```python
from build123d import *

# Parameters (mm, degrees)
SKETCH2_W           = 98
SKETCH2_H           = 42
SKETCH2_R           = 6
BOSS_EXTRUDE1_DEPTH = 20
SKETCH3_W           = 70
SKETCH3_H           = 6
CUT_EXTRUDE2_DEPTH  = 20
SKETCH4_W           = 70
SKETCH4_H           = 6
CUT_EXTRUDE3_DEPTH  = 20
SKETCH5_W           = 4.083920217
SKETCH5_H           = 6
CUT_EXTRUDE4_DEPTH  = 20
SKETCH6_W           = 4.083920217
SKETCH6_H           = 6
CUT_EXTRUDE5_DEPTH  = 20
SKETCH7_W           = 38.167840434
SKETCH7_H           = 6
CUT_EXTRUDE6_DEPTH  = 20
SKETCH8_R           = 10
BOSS_EXTRUDE2_DEPTH = 7
FILLET2_R           = 5
FILLET3_R           = 10


with BuildPart() as part:
    # Sketch2 → Boss-Extrude1 (new body)
    with BuildSketch(Plane(origin=(0, 0, 0), x_dir=(1, 0, 0), z_dir=(0, 1, 0))):
        Rectangle(SKETCH2_W, SKETCH2_H)
        with Locations((25, 0)):
            Circle(SKETCH2_R, mode=Mode.SUBTRACT)
        with Locations((-25, 0)):
            Circle(SKETCH2_R, mode=Mode.SUBTRACT)
    extrude(amount=-BOSS_EXTRUDE1_DEPTH)

    # Sketch3 → Cut-Extrude2 (cut)
    with BuildSketch(Plane.XY.offset(21)):
        with Locations((0, -17)):
            Rectangle(SKETCH3_W, SKETCH3_H)
    extrude(amount=-CUT_EXTRUDE2_DEPTH, mode=Mode.SUBTRACT)

    # Sketch4 → Cut-Extrude3 (cut)
    with BuildSketch(Plane(origin=(0, 0, -21), x_dir=(-1, 0, 0), z_dir=(0, 0, -1))):
        with Locations((0, -17)):
            Rectangle(SKETCH4_W, SKETCH4_H)
    extrude(amount=-CUT_EXTRUDE3_DEPTH, mode=Mode.SUBTRACT)

    # Sketch5 → Cut-Extrude4 (cut)
    with BuildSketch(Plane.XY.offset(1)):
        with Locations((32.958039892, -17)):
            Rectangle(SKETCH5_W, SKETCH5_H)
    extrude(amount=-CUT_EXTRUDE4_DEPTH, mode=Mode.SUBTRACT)

    # Sketch6 → Cut-Extrude5 (cut)
    with BuildSketch(Plane.XY.offset(1)):
        with Locations((-32.958039892, -17)):
            Rectangle(SKETCH6_W, SKETCH6_H)
    extrude(amount=-CUT_EXTRUDE5_DEPTH, mode=Mode.SUBTRACT)

    # Sketch7 → Cut-Extrude6 (cut)
    with BuildSketch(Plane.XY.offset(1)):
        with Locations((0, -17)):
            Rectangle(SKETCH7_W, SKETCH7_H)
    extrude(amount=-CUT_EXTRUDE6_DEPTH, mode=Mode.SUBTRACT)

    # Sketch8 → Boss-Extrude2 (add, symmetric)
    with BuildSketch(Plane.ZY):
        with BuildLine():
            Line((-21, 0), (21, 0))
            Line((21, 0), (21, 21))
            ThreePointArc((21, 21), (0, 42), (-21, 21))
            Line((-21, 21), (-21, 0))
        make_face()
        with Locations((0, 21)):
            Circle(SKETCH8_R, mode=Mode.SUBTRACT)
    extrude(amount=BOSS_EXTRUDE2_DEPTH, both=True)

    # Fillet2
    fillet2_edges = [part.edges().sort_by_distance(p)[0] for p in [
        (-7, 0, 0),
    ]]
    fillet(fillet2_edges, radius=FILLET2_R)

    # Fillet3
    fillet3_edges = [part.edges().sort_by_distance(p)[0] for p in [
        (7, 0, 0),
        (-49, 0, 0),
        (49, 0, 0),
    ]]
    fillet(fillet3_edges, radius=FILLET3_R)


solid = part.part
```
Design review of the part built by this model. Coordinates are the model's own, in mm. A direction names the side the tool comes from. Round coordinates to 2 decimals unless told otherwise and drop trailing zeros. Write each loop counter-clockwise with the first axis right and the second up, starting at its lowest first coordinate (ties: lowest second). Pieces come first, ordered by that corner, then holes.
Item 1: For probe 1 along X at (y, z) = (-9.5, 0); probe 2 along Z at (x, y) = (-25, -7); probe 3 along Y at (x, z) = (3, 0), list the stretches that pass through material, from the lowest coordinate up.
Item 2: We need section B-B on y = 15. Write out the cut boundary in (x, z).
Item 3: For faces 1 (the cylindrical face through (20.24, -6.9, 3.65)), 2 (the flat face through (-7, 24, -10)), 3 (the flat face through (-1, -4, -21)), 4 (the flat face through (7, 30, -5)), 5 (the flat face through (0, -14, 0)), list the 3-axis set-ups (+Z, -Z, +X, -X, +Y, -Y) from which the entire face can be reached by the end or side of a thin tool; tool diameter is ignored.
Item 4: Clearance check with flat-ended pins moving along their axes: pin 1 Ø10 at (x, z) = (-4.5, 1.5) entering from -Y; pin 2 Ø2 at (y, z) = (13, 14.5) entering from +X; pin 3 Ø6.5 at (x, z) = (31.5, -7.5) entering from +Y. State where each tip first meets the part, or that it passes through.
Item 5: We need section A-A on x = -25. Write out the cut boundary in (y, z).
Item 6: The part is to be moulded in two halves that separate along X. For faces 6 (the flat face through (49, -15, 0)), 7 (the cylindrical face through (-29.76, -6.9, 3.65)), 8 (the cylindrical face through (0, 42, 0)), say which applies: +X half, -X half, draft (parallel to the pull), parting line (faces both ways), or undercut.
Item 7: We need section C-C on z = 2. Write out the cut boundary in (x, y), and give its area (3 significant figures).
Item 8: We need section D-D on z = 9. Write out the cut boundary in (x, y).
Returned:
1. probe 1: x = -48.99 to -31, -19 to 19, 31 to 48.99
1. probe 2: z = -21 to -6, 6 to 21
1. probe 3: y = -14 to 11, 31 to 42
2. outline: (-7, -21) - (7, -21) - (7, -8) - (-7, -8) - close; (-7, 8) - (7, 8) - (7, 21) - (-7, 21) - close
3. face 1: +Y, -Y
3. face 2: +Z, -Z, -X, +Y
3. face 3: -Z, +X, -X, +Y, -Y
3. face 4: +Z, -Z, +X, +Y
3. face 5: +Z, -Z, -Y
4. pin 1: stops at y = -14
4. pin 2: stops at x = 7
4. pin 3: stops at y = 0
5. outline: (-14, -21) - (0, -21) - (0, -6) - (-14, -6) - close; (-14, 6) - (0, 6) - (0, 21) - (-14, 21) - close
6. face 6: +X half
6. face 7: undercut
6. face 8: draft
7. outline: (-49, -20) - (-35, -20) - (-35, -14) - (-30.66, -14) - (-30.66, 0) - (-39, 0) arc R10 ccw to (-49, -10) - close; (-19.34, -14) - (19.34, -14) - (19.34, 0) - (17, 0) arc R10 cw to (7, 10) - (7, 11.2) - (-7, 11.2) - (-7, 5) arc R5 cw to (-12, 0) - (-19.34, 0) - close; (-7, 30.8) - (7, 30.8) - (7, 41.9) - (-7, 41.9) - close; (30.66, -14) - (35, -14) - (35, -20) - (49, -20) - (49, -10) arc R10 ccw to (39, 0) - (30.66, 0) - close
7. area: 1,520 mm2
8. outline: (-49, -20) - (-35, -20) - (-35, -14) - (35, -14) - (35, -20) - (49, -20) - (49, -10) arc R10 ccw to (39, 0) - (17, 0) arc R10 cw to (7, 10) - (7, 16.64) - (-7, 16.64) - (-7, 5) arc R5 cw to (-12, 0) - (-39, 0) arc R10 ccw to (-49, -10) - close; (-7, 25.36) - (7, 25.36) - (7, 39.97) - (-7, 39.97) - close
